Autodesk Inventor part; units mm, degrees
ref_plane "YZ Plane" through (0, 0, 0) normal (1, 0, 0) x (0, 1, 0)
ref_plane "XZ Plane" through (0, 0, 0) normal (0, 1, 0) x (-1, 0, 0)
ref_plane "XY Plane" through (0, 0, 0) normal (0, 0, 1) x (1, 0, 0)
sketch "Sketch1" plane through (0, 0, 0) normal (1, 0, 0) x (0, 1, 0)
  line L0 (12.7439, 15.061) -> (-12.2561, 15.061)
  line L1 (-12.2561, 15.061) -> (-12.2561, -9.939)
  line L2 (-12.2561, -9.939) -> (12.7439, -9.939)
  line L3 (12.7439, -9.939) -> (12.7439, 15.061)
  point P0 (0, 0)
  dimension "d0" = 25
  dimension "d1" = 25
extrude "Extrusion1" add sketch "Sketch1" along normal blind 6
fillet "Fillet1" radius 2 4 edges at (3, -12.2561, 15.061) (3, 12.7439, 15.061) (3, -12.2561, -9.939) (3, 12.7439, -9.939)
sketch "Sketch2" plane through (0, 0, 0) normal (-1, 0, 0) x (0, 0, 1)
  circle A0 centre (12.561, 10.2439) radius 1.25
  circle A1 centre (12.561, -9.7561) radius 1.25
  circle A2 centre (-7.439, -9.7561) radius 1.25
  circle A3 centre (-7.439, 10.2439) radius 1.25
  line L0 (15.061, 10.7439) -> (15.061, -10.2561)
  line L1 (-7.939, 12.7439) -> (13.061, 12.7439)
  line L2 (13.061, -12.2561) -> (-7.939, -12.2561)
  line L3 (-9.939, -10.2561) -> (-9.939, 10.7439)
  point P0 (0, 0)
  dimension "d5" = 2.5
  dimension "d6" = 2.5
  dimension "d7" = 2.5
  dimension "d8" = 2.5
  dimension "d9" = 2.5
  dimension "d10" = 2.5
  dimension "d11" = 2.5
  dimension "d12" = 2.5
  dimension "d13" = 2.5
  dimension "d14" = 2.5
  dimension "d15" = 2.5
  dimension "d16" = 2.5
extrude "Extrusion2" cut sketch "Sketch2" against normal through all
sketch "Sketch3" plane through (0, 0, 0) normal (-1, 0, 0) x (0, 0, 1)
  circle A0 centre (2.561, 0.2439) radius 5
  line L0 (13.061, -12.2561) -> (-7.939, -12.2561)
  line L1 (15.061, 10.7439) -> (15.061, -10.2561)
  point P0 (0, 0)
  dimension "d19" = 10
  dimension "d20" = 12.5
  dimension "d21" = 12.5
extrude "Extrusion3" cut sketch "Sketch3" against normal blind 10
properties part number "25mmx25mmx6mm_fan"
Can you work these out from the model? Positions are in its coordinate system, mm. Coordinates: 2 decimals unless noted, no trailing zeros. Order: outer loops, then holes, each group sorted by start corner. A loop starts at its lowest first (then second) coordinate and runs counter-clockwise, first axis right, second up. Notation, with made-up numbers: (58.5, 79) - (96.5, 79) arc R16 ccw to (96.5, 100) - close; hole circle Ø11 at (-29.5, 12). An arc over 180 degrees is marked (long way). Answer in a Markdown table with one row per item.
1. If we mould it in two halves opening along Y, with no side actions, what happens to faces 1 (the flat face through (3, 12.744, 2)), 2 (the cylindrical face through (2.96, -8.7, 13.23)), 3 (the flat face through (3, 0, 15.061)), 4 (the flat face through (3, -12.256, 3))? For each: pulls with the +Y half, pulls with the -Y half, needs draft (parallel to the pull), parting line crosses it, or undercut.
Reply:
| item | result |
|---|---|
| face 1 | pulls with the +Y half |
| face 2 | undercut |
| face 3 | needs draft |
| face 4 | pulls with the -Y half |
2. If I drill on line 1 along Z through (x, y) = (1.3, -9.25); line 2 along Y through (x, z) = (3.95, 5.75); line 3 along Y through (x, z) = (3.1, -1.75), over which ranges is the centre line in solid material (lowest first)?
Reply:
| item | result |
|---|---|
| line 1 | z = -9.94 to -8.58, -6.3 to 11.42, 13.7 to 15.06 |
| line 2 | y = -12.26 to -3.61, 4.09 to 12.74 |
| line 3 | y = -12.26 to -2.29, 2.78 to 12.74 |
3. Suppose I cut it at A-A (z = 3.75). Please give me the cut outline in (x, y).
Reply:
| item | result |
|---|---|
| outline | (0, -12.26) - (6, -12.26) - (6, -4.61) - (0, -4.61) - close; (0, 5.1) - (6, 5.1) - (6, 12.74) - (0, 12.74) - close |
4. Suppose I cut it at C-C (x = 3.2). Please give me the cut outline in (y, z), and give its area (3 significant figures).
Reply:
| item | result |
|---|---|
| outline | (-12.26, -7.94) arc R2 ccw to (-10.26, -9.94) - (10.74, -9.94) arc R2 ccw to (12.74, -7.94) - (12.74, 13.06) arc R2 ccw to (10.74, 15.06) - (-10.26, 15.06) arc R2 ccw to (-12.26, 13.06) - close; hole circle Ø2.5 at (-9.76, -7.44); hole circle Ø2.5 at (-9.76, 12.56); hole circle Ø10 at (0.24, 2.56); hole circle Ø2.5 at (10.24, -7.44); hole circle Ø2.5 at (10.24, 12.56) |
| area | 523 mm^2 |
5. Suppose I cut it at B-B (y = -0.5). Please give me the cut outline in (x, z), and give its area (3 significant figures).
Reply:
| item | result |
|---|---|
| outline | (0, -9.94) - (6, -9.94) - (6, -2.38) - (0, -2.38) - close; (0, 7.51) - (6, 7.51) - (6, 15.06) - (0, 15.06) - close |
| area | 90.7 mm^2 |
